```python
from build123d import *

# Parameters (mm, degrees)
SKETCH1_R           = 1.5
SKETCH1_R_2         = 2.4
BOSS_EXTRUDE1_DEPTH = 6


with BuildPart() as part:
    # Sketch1 → Boss-Extrude1 (new body)
    with BuildSketch(Plane(origin=(0, 0, 0), x_dir=(1, 0, 0), z_dir=(0, 1, 0))):
        with BuildLine():
            Line((-19.436129881, 35.921169676), (-20.784472899, 19.250484474))
            ThreePointArc((-20.784472899, 19.250484474), (-17.739772521, 8.917849876), (-8.554847577, 3.290177898))
            Line((-8.554847577, 3.290177898), (8.303819749, 0.179771806))
            ThreePointArc((8.303819749, 0.179771806), (10.722077148, -2.298002723), (9.194413259, -5.405023565))
            Line((9.194413259, -5.405023565), (-40.652031907, -32.553428604))
            ThreePointArc((-40.652031907, -32.553428604), (-42.651504917, -39.335913966), (-35.869019555, -41.335386976))
            Line((-35.869019555, -41.335386976), (31.012382829, -4.909050143))
            ThreePointArc((31.012382829, -4.909050143), (33.55848931, 0.269317926), (29.528060312, 4.398942141))
            Line((29.528060312, 4.398942141), (-7.891068482, 11.302731386))
            ThreePointArc((-7.891068482, 11.302731386), (-10.95271013, 13.178622045), (-11.967610256, 16.622833578))
            Line((-11.967610256, 16.622833578), (-10.465424103, 35.195609308))
            ThreePointArc((-10.465424103, 35.195609308), (-14.587996808, 40.043742381), (-19.436129881, 35.921169676))
        make_face()
        with Locations((28.620876654, -0.518070957)):
            Circle(SKETCH1_R, mode=Mode.SUBTRACT)
        with Locations((-14.950776992, 35.558389492)):
            Circle(SKETCH1_R_2, mode=Mode.SUBTRACT)
    extrude(amount=BOSS_EXTRUDE1_DEPTH)


solid = part.part
```
Could you check a few things on this model? Use its own coordinates, in mm. A direction names the side the tool comes from. Round coordinates to 2 decimals unless told otherwise and drop trailing zeros. Loops run counter-clockwise (first coordinate to the right, second up) from the corner with the lowest first, then second, coordinate; pieces in that order, holes last. Notation, with made-up numbers: M 31,16.5 L 83,16.5 A4 cw 83,22.5 Z; hole C 0.5,64 d1. An arc over 180 degrees is marked long. Put each result on its own line as item: value.
Q1. For pin 1 (7.5 mm diameter, centred on x = -14.95, z = -35.56, fed in from +Y); pin 2 (2 mm diameter, centred on y = 1.5, z = 31, fed in from +X); pin 3 (2 mm diameter, centred on y = 2, z = -21, fed in from -X), each with a flat end and sliding along its axis, tell me the tip position at first contact or that it passes through.
Check result:
pin 1: y = 6
pin 2: x = -15.06
pin 3: x = -20.72
Q2. Imagine slicing it at B-B (z = 35.5). Write out the boundary of the cut face in (x, y).
Check result:
outline: M -43.05,0 L -25.15,0 L -25.15,6 L -43.05,6 Z
Q3. On a 3-axis mill with a long thin cutter (end or side, diameter ignored), from which of +Z, -Z, +X, -X, +Y, -Y can I reach the whole of each face in a straight line? I mean faces 1 (the face through (-15.4, 3, 18.8)), 2 (the face through (-11.227, 2.958, -25.779)), 3 (the face through (30.052, 2.958, 0.068)). Say none if no direction works.
Check result:
face 1: -X, +Y, -Y
face 2: +X, +Y, -Y
face 3: +Y, -Y
Q4. Imagine slicing it at A-A (y = 5.1). Write out the boundary of the cut face in (x, z), then the cut area to 3 significant figures.
Check result:
outline: M -40.65,32.55 L 9.19,5.41 A3 cw 8.3,-0.18 L -8.55,-3.29 A15 ccw -20.78,-19.25 L -19.44,-35.92 A4.5 ccw -10.47,-35.2 L -11.97,-16.62 A5 cw -7.89,-11.3 L 29.53,-4.4 A5 ccw 31.01,4.91 L -35.87,41.34 A5 ccw Z; hole C -14.95,-35.56 d4.8; hole C 28.62,0.52 d3
area: 1,390 mm2
Q5. I need wall thicknesses on probe 1 along Z at (x, y) = (-14, 4.55); probe 2 along Z at (x, y) = (-1.5, 5.5); probe 3 along Z at (x, y) = (-1, 0.55). Which ranges of each line are inside material? Lowest first, please.
Check result:
probe 1: -39.96 to -37.76, -33.35 to -5.46, 18.04 to 29.42
probe 2: -10.12 to -1.99, 11.23 to 22.62
probe 3: -10.03 to -1.9, 10.96 to 22.34
Q6. Imagine slicing it at C-C (x = -23.5). Write out the boundary of the cut face in (y, z).
Check result:
outline: M 0,23.21 L 6,23.21 L 6,34.6 L 0,34.6 Z
Q7. Thinking about a two-plate mould opening in Z: for faces 4 (the face through (-20.1, 3, -27.7)), 5 (the face through (-0.244, 2.958, -1.757)), 6 (the face through (-2, 6, 13)), which applies, released by +Z, released by -Z, zero draft, split by the parting line, or undercut?
Check result:
face 4: released by -Z
face 5: undercut
face 6: zero draft
